Could you check a few things on this model? Use its own coordinates, in mm. Face numbers are marked on the shaded views. A direction names the side the tool comes from. Give positions to 0.01 mm unless a question says otherwise; leave off trailing zeros. Order: outer loops, then holes, each group sorted by start corner. A loop starts at its lowest first (then second) coordinate and runs counter-clockwise, first axis right, second up. Notation, with made-up numbers: M 88,-12 L 109,-12 A17 cw 109,-5 Z; hole C -37.5,30.5 d1. An arc over 180 degrees is marked long. Use a Markdown table: item, result. Add a question column.
```python
from build123d import *

# Parameters (mm, degrees)
SKETCH_1_W          = 18
SKETCH_1_H          = 33.5
EXTRUDE_1_DEPTH     = 12
SHELL_1_T           = -1.5
FILLET_1_R          = 1.5
SKETCH_2_W          = 15
SKETCH_2_H          = 5.3
EXTRUDE_2_DEPTH     = 2.5
SKETCH_4_W          = 6
SKETCH_4_H          = 2.5
CUT_EXTRUDE_1_DEPTH = 2.5
FILLET_3_R          = 1.5
SKETCH_5_W          = 9
SKETCH_5_H          = 3.4
CUT_EXTRUDE_2_DEPTH = 2.5
SKETCH_6_W          = 12
SKETCH_6_H          = 8
CUT_EXTRUDE_3_DEPTH = 2.5
SKETCH_7_R          = 0.9
CUT_EXTRUDE_4_DEPTH = 3
SKETCH_8_R          = 0.9
CUT_EXTRUDE_5_DEPTH = 23.5
SKETCH_10_R         = 2
CUT_EXTRUDE_7_DEPTH = 0.75
CUT_EXTRUDE_START   = -0.75
SKETCH_11_R         = 2
CUT_EXTRUDE_8_DEPTH = 0.75


with BuildPart() as part:
    # 草图1 → 凸台-拉伸1 (new body)
    with BuildSketch(Plane(origin=(0, 0, 0), x_dir=(1, 0, 0), z_dir=(0, 1, 0))):
        Rectangle(SKETCH_1_W, SKETCH_1_H)
    extrude(amount=EXTRUDE_1_DEPTH)

    # 抽壳1
    shell_1_openings = [part.faces().sort_by_distance(p)[0] for p in [
        (0, 12, 0),
    ]]
    offset(amount=SHELL_1_T, openings=shell_1_openings, kind=Kind.INTERSECTION)

    # 圆角1
    fillet_1_edges = [part.edges().sort_by_distance(p)[0] for p in [
        (0, 0, -16.75),
        (9, 0, 0),
        (0, 0, 16.75),
        (-9, 0, 0),
        (-9, 6, -16.75),
        (9, 6, -16.75),
        (9, 6, 16.75),
        (-9, 6, 16.75),
    ]]
    fillet(fillet_1_edges, radius=FILLET_1_R)

    # 草图2 → 凸台-拉伸2 (add)
    with BuildSketch(Plane(origin=(0, 1.5, 0), x_dir=(1, 0, 0), z_dir=(0, 1, 0))):
        with Locations((0, -12.6)):
            Rectangle(SKETCH_2_W, SKETCH_2_H)
    extrude(amount=EXTRUDE_2_DEPTH)

    # 草图4 → 切除-拉伸1 (cut)
    with BuildSketch(Plane(origin=(0, 4, 0), x_dir=(1, 0, 0), z_dir=(0, 1, 0))):
        with Locations((-1.5, -11.2)):
            Rectangle(SKETCH_4_W, SKETCH_4_H)
    extrude(amount=-CUT_EXTRUDE_1_DEPTH, mode=Mode.SUBTRACT)

    # 圆角3
    fillet_3_edges = [part.edges().sort_by_distance(p)[0] for p in [
        (4.5, 1.5, 9.95),
        (-6, 1.5, 9.95),
    ]]
    fillet(fillet_3_edges, radius=FILLET_3_R)

    # 草图5 → 切除-拉伸2 (cut)
    with BuildSketch(Plane(origin=(0, 0, 15.25), x_dir=(-1, 0, 0), z_dir=(0, 0, -1))):
        with Locations((1.3, 6.9)):
            Rectangle(SKETCH_5_W, SKETCH_5_H)
    extrude(amount=-CUT_EXTRUDE_2_DEPTH, mode=Mode.SUBTRACT)

    # 草图6 → 切除-拉伸3 (cut)
    with BuildSketch(Plane(origin=(0, 0, -16.75), x_dir=(-1, 0, 0), z_dir=(0, 0, -1))):
        with Locations((0, 9.1)):
            Rectangle(SKETCH_6_W, SKETCH_6_H)
    extrude(amount=-CUT_EXTRUDE_3_DEPTH, mode=Mode.SUBTRACT)

    # 草图7 → 切除-拉伸4 (cut)
    with BuildSketch(Plane(origin=(0, 4, 0), x_dir=(1, 0, 0), z_dir=(0, 1, 0))):
        with Locations(Location((5.3, -11.55, 0), (0, 0, 270))):
            Circle(SKETCH_7_R)
    extrude(amount=-CUT_EXTRUDE_4_DEPTH, mode=Mode.SUBTRACT)

    # 草图8 → 切除-拉伸5 (cut)
    with BuildSketch(Plane(origin=(9, 0, 0), x_dir=(0, 0, -1), z_dir=(1, 0, 0))):
        with Locations((-3.25, 8)):
            Circle(SKETCH_8_R)
    extrude(amount=-CUT_EXTRUDE_5_DEPTH, mode=Mode.SUBTRACT)

    # 草图10 → 切除-拉伸7 (cut)
    with BuildSketch(Plane(origin=(9, 0, 0), x_dir=(0, 0, -1), z_dir=(1, 0, 0))):
        with Locations((-3.25, 8)):
            Circle(SKETCH_10_R)
    extrude(amount=-CUT_EXTRUDE_7_DEPTH, mode=Mode.SUBTRACT)

    # 草图11 → 切除-拉伸8 (cut)
    with BuildSketch(Plane.ZY.offset(9).offset(CUT_EXTRUDE_START)):
        with Locations(Location((3.25, 8, 0), (0, 0, 180))):
            Circle(SKETCH_11_R)
    extrude(amount=CUT_EXTRUDE_8_DEPTH, mode=Mode.SUBTRACT)


solid = part.part
```
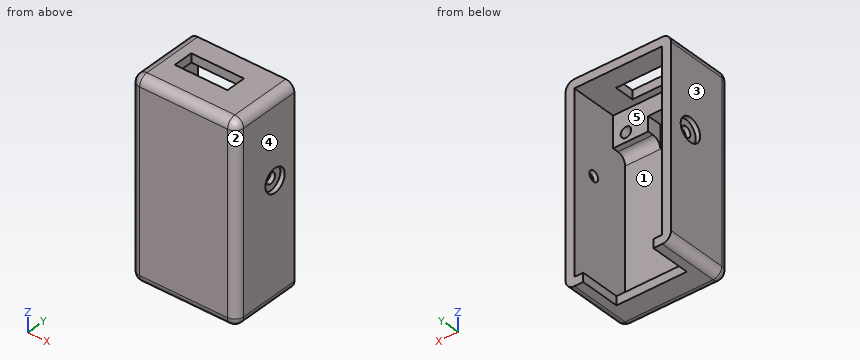
1) For pin 1 (0.5 mm diameter, centred on x = 5.5, z = 11.5, fed in from +Y); pin 2 (4 mm diameter, centred on x = 4, z = -3, fed in from +Y); pin 3 (1.1 mm diameter, centred on y = 8, z = 3.25, fed in from +X), each with a flat end and sliding along its axis, tell me the tip position at first contact or that it passes through.
2) We'd pull the mould along X, two halves only. Please class the marked faces 3, 4 and 5: pulls with the +X half, pulls with the -X half, needs draft (parallel to the pull), parting line crosses it, or undercut.
3) Suppose I cut it at A-A on x = -4. Please give me the cut outline in (y, z), and give its area (3 significant figures).
4) Suppose I cut it at C-C on y = 8. Count the separate pieces of the cut face and the enclosed holes in it, and give its area (3 significant figures).
5) Suppose I cut it at B-B on z = 3.25. Please give me the cut outline in (x, y).
6) Please list where these lines run through material, in increasing order: line 1 (X direction, y = 2.2, z = 11.55); line 2 (X direction, y = 8.5, z = -14); line 3 (Z direction, x = 4.5, y = 2). Write a range as from..to.
7) For the marked faces 1 and 2, which set-ups out of +Z, -Z, +X, -X, +Y, -Y let a thin tool reach every point of the face, with its end or its side?
8) Suppose I cut it at D-D on z = -9. Please give me the cut outline in (x, y), and give its area (3 significant figures).
Values found:
| question | item | result |
|---|---|---|
| 1 | pin 1 | stops at y = 1 |
| 1 | pin 2 | stops at y = 1.5 |
| 1 | pin 3 | passes through |
| 2 | face 3 | pulls with the -X half |
| 2 | face 4 | pulls with the +X half |
| 2 | face 5 | undercut |
| 3 | outline | M 0,-15.25 A1.5 ccw 1.5,-16.75 L 5.1,-16.75 L 5.1,-15.25 L 1.5,-15.25 L 1.5,12.45 L 4,12.45 L 4,15.25 L 5.2,15.25 L 5.2,16.75 L 1.5,16.75 A1.5 ccw 0,15.25 Z; M 8.6,15.25 L 12,15.25 L 12,16.75 L 8.6,16.75 Z |
| 3 | area | 72.3 mm^2 |
| 4 | separate pieces | 4 |
| 4 | enclosed holes | 0 |
| 4 | area | 103 mm^2 |
| 5 | outline | M -9,1.5 A1.5 ccw -7.5,0 L 7.5,0 A1.5 ccw 9,1.5 L 9,6 L 8.25,6 L 8.25,7.1 L 7.5,7.1 L 7.5,1.5 L -7.5,1.5 L -7.5,7.1 L -8.25,7.1 L -8.25,6 L -9,6 Z; M -9,10 L -8.25,10 L -8.25,8.9 L -7.5,8.9 L -7.5,12 L -9,12 Z; M 7.5,8.9 L 8.25,8.9 L 8.25,10 L 9,10 L 9,12 L 7.5,12 Z |
| 6 | line 1 | x = -9..-4.5, 1.5..4.4, 6.2..9 |
| 6 | line 2 | x = -9..-7.5, 7.5..9 |
| 6 | line 3 | z = -16.75..-15.25, 9.57..11.14, 11.96..16.75 |
| 7 | face 1 | +Y |
| 7 | face 2 | +Z, -Z, +X, -Y |
| 8 | outline | M -9,1.5 A1.5 ccw -7.5,0 L 7.5,0 A1.5 ccw 9,1.5 L 9,12 L 7.5,12 L 7.5,1.5 L -7.5,1.5 L -7.5,12 L -9,12 Z |
| 8 | area | 57.5 mm^2 |
